Autodesk Inventor part; units mm, degrees
ref_plane "YZ Plane" through (0, 0, 0) normal (1, 0, 0) x (0, 1, 0)
ref_plane "XZ Plane" through (0, 0, 0) normal (0, 1, 0) x (-1, 0, 0)
ref_plane "XY Plane" through (0, 0, 0) normal (0, 0, 1) x (1, 0, 0)
sketch "Sketch1" plane through (0, 0, 0) normal (0, 0, 1) x (1, 0, 0)
  arc A0 (17, 50.9482) -> (0, 53.5) centre (-5.1444, -38.6736) ccw
  arc A1 (34.618, 33) -> (17, 50.9482) centre (11.2519, 27.6848) ccw
  arc A2 (36, 0) -> (34.618, 33) centre (-54.4409, 12.7413) ccw
  line L0 (36, 0) -> (36, -81) construction
  arc A3 (-50, 0) -> (-47.876, -9) centre (-23.2557, 1.561) ccw
  line L1 (-50, 0) -> (-52.0013, -78) construction
  arc A4 (-39.1762, -46) -> (-47.876, -9) centre (-148.6013, -52.2064) ccw
  arc A5 (-48.0013, -70.0072) -> (-39.1762, -46) centre (-76.244, -45.9995) ccw
  arc A6 (-48.0013, -70.0072) -> (-52.0013, -78) centre (-33.7069, -82.1582) ccw
  line L2 (36, 0) -> (36, -81) construction
  arc A7 (0, 53.5) -> (-50, 0) centre (-4.0952, 7.2128) ccw
  arc A8 (-52.0013, -78) -> (-50.4909, -84.4368) centre (-45.2921, -79.8213) ccw
  arc A9 (-50.4909, -84.4368) -> (-25.5013, -104) centre (5.8002, -38.274) ccw
  line L3 (-25.5013, -104) -> (18, -104)
  arc A10 (36, 0) -> (33.2377, -67.2753) centre (254.1506, -42.6516) ccw
  arc A11 (18, -104) -> (35.9231, -85.173) centre (7.7888, -76.3343) ccw
  arc A12 (33.2377, -67.2753) -> (36, -81) centre (112.7493, -58.4127) ccw
  arc A13 (35.9231, -85.173) -> (36, -81) centre (29.326, -82.9642) ccw
  point P0 (0, 0)
  dimension "d6" = 53.5
  dimension "d7" = 50
  dimension "d8" = 36
  dimension "d10" = 81
  dimension "d16" = 78
  dimension "d18" = 9
  dimension "d24" = 4
  dimension "d28" = 33
  dimension "d29" = 46
  dimension "d33" = 104
  dimension "d34" = 26.5
  dimension "d35" = 18
  dimension "d36" = 0
  dimension "d38" = 92.317
  dimension "d39" = 91.334
  dimension "d40" = 46.468
  dimension "d41" = 26.7899
  dimension "d42" = 222.281
  dimension "d43" = 80.004
  dimension "d44" = 109.601
  dimension "d45" = 37.0678
  dimension "d46" = 18.761
  dimension "d47" = 6.952
  dimension "d48" = 72.799
  dimension "d49" = 29.49
  dimension "d50" = 6.957
  dimension "d51" = 17
  dimension "d52" = 0
  dimension "d53" = 23.963
  dimension "d54" = 50
  dimension "d55" = 2.0013
  dimension "d56" = 12.0001
  dimension "d57" = 67.2753
  dimension "d58" = 18.827
  dimension "d59" = 19.5632
  dimension "d61" = 24.9896
extrude "Extrusion1" add sketch "Sketch1" along normal blind 2
properties part number "_3DPrint"
Geometry: final body of the model. Coordinates: model frame, mm. A direction names the side the tool comes from. Round coordinates to 2 decimals unless told otherwise and drop trailing zeros. Loops run counter-clockwise (first coordinate to the right, second up) from the corner with the lowest first, then second, coordinate; pieces in that order, holes last. Notation, with made-up numbers: (2.25, 41.5) -> (43.25, 41.5) arc R33 cw to (43.25, 71.5) -> close; hole circle Ø11 at (18.25, 63). An arc over 180 degrees is marked (long way). Use one line per item in the form item = value. Start each with the question number.
1) Section A-A on x = -44. Output: boundary loops of the cut face in (y, z), then the cut area to 3 significant figures.
2) Section C-C on y = -88. Output: boundary loops of the cut face in (x, z), then the cut area to 3 significant figures.
3) Section D-D on x = -30. Output: boundary loops of the cut face in (y, z), then the cut area to 3 significant figures.
4) Section B-B on z = 0.8. Output: boundary loops of the cut face in (x, y).
5) First-contact query: P1, Ø1, axis at y = 26, z = 1, coming from the -X side. Flat tip, straight axial feed; report the tip coordinate or a pass-through.
6) Access query for faces 4 (the cylindrical face through (28.223, 44.603, 0.986)), 5 (the cylindrical face through (-50.512, -73.818, 0.986)), 6 (the cylindrical face through (34.337, -74.294, 0.986)). Directions: +Z, -Z, +X, -X, +Y, -Y. A direction counts if a zero-diameter tool reaches every point of the face in a straight line with its end or side. Return the directions, or none.
7) Line query: L1, parallel to X at y = -0.5, z = 1.3; L2, parallel to Y at x = -25.5, z = 0.55; L3, parallel to Y at x = -3.5, z = 1.05. Output: solid intervals per line, ascending.
8) Draft query along Y for faces 1 (the cylindrical face through (-41.39, -58.62, 0.99)), 2 (the flat face through (-8, -24, 0)), 3 (the cylindrical face through (-38.899, -95.735, 0.986)). Return one class per face: released by +Y, released by -Y, zero draft, split by the parting line, or undercut.
Response:
q1.outline = (-91.37, 0) -> (-64.28, 0) -> (-64.28, 2) -> (-91.37, 2) -> close; (-19.48, 0) -> (31.02, 0) -> (31.02, 2) -> (-19.48, 2) -> close
q1.area = 155 mm^2
q2.outline = (-47.37, 0) -> (34.87, 0) -> (34.87, 2) -> (-47.37, 2) -> close
q2.area = 164 mm^2
q3.outline = (-101.66, 0) -> (45.79, 0) -> (45.79, 2) -> (-101.66, 2) -> close
q3.area = 295 mm^2
q4.outline = (-52, -78) arc R6.95 ccw to (-50.49, -84.44) arc R72.8 ccw to (-25.5, -104) -> (18, -104) arc R29.49 ccw to (35.92, -85.17) arc R6.96 ccw to (36, -81) arc R80 cw to (33.24, -67.28) arc R222.28 cw to (36, 0) arc R91.33 ccw to (34.62, 33) arc R23.96 ccw to (17, 50.95) arc R92.31 ccw to (0, 53.5) arc R46.47 ccw to (-50, 0) arc R26.79 ccw to (-47.88, -9) arc R109.6 cw to (-39.18, -46) arc R37.07 cw to (-48, -70.01) arc R18.76 ccw to start
q5.P1 = -46.81
q6.face_4 = +Z, -Z, +X, +Y
q6.face_5 = +Z, -Z, -X
q6.face_6 = +Z, -Z, +X
q7.L1 = -49.97 to 35.9
q7.L2 = -104 to 48.46
q7.L3 = -104 to 53.68
q8.face_1 = undercut
q8.face_2 = zero draft
q8.face_3 = released by -Y
